Geometry: final body of the model. Coordinates: model frame, mm. A direction names the side the tool comes from. Coordinates: 2 decimals unless noted, no trailing zeros. Write each loop counter-clockwise with the first axis right and the second up, starting at its lowest first coordinate (ties: lowest second). Pieces come first, ordered by that corner, then holes. Notation, with made-up numbers: (-20, 89.25) - (38, 89.25) arc R12 ccw to (38, 96.25) - close; hole circle Ø2 at (5.25, 4). An arc over 180 degrees is marked (long way). Put each result on its own line as item: value.
```python
from build123d import *

# Parameters (mm, degrees)
F1_DEPTH  = 21
F2_W      = 22
F2_H      = 21
F3_DEPTH  = 4
F4_R      = 6.6
F4_R_2    = 1.35
F5_DEPTH  = 17.501
F6_R      = 1.8
F7_DEPTH  = 7
F8_R      = 4
F9_DEPTH  = 3
F10_R     = 1.35
F11_DEPTH = 12


# Not quite as in the source:
# - a feature names something its author has since deleted; it is built from what else it names


with BuildPart() as f1:
    # F0 (on Front) → F1 (new body)
    with BuildSketch(Plane.XZ):
        with BuildLine():
            Line((-9, -2.5), (-6.5, 0))
            Line((-6.5, 0), (-11, 0))
            Line((-11, 0), (-11, -5))
            Line((-11, -5), (-6.5, -5))
            Line((-6.5, -5), (-6.5, -39))
            Line((-6.5, -39), (6.5, -39))
            Line((6.5, -39), (6.5, -5))
            Line((6.5, -5), (11, -5))
            Line((11, -5), (11, 0))
            Line((11, 0), (6.5, 0))
            Line((6.5, 0), (9, -2.5))
            Line((9, -2.5), (0.75, -2.5))
            Line((0.75, -2.5), (0.75, -17.11916493))
            ThreePointArc((0.75, -17.11916493), (0, -20.9732145518), (-0.75, -17.11916493))
            Line((-0.75, -17.11916493), (-0.75, -2.5))
            Line((-0.75, -2.5), (-9, -2.5))
        make_face()
    extrude(amount=F1_DEPTH)

    # F2 (on face) → F3 (cut)
    with BuildSketch(Plane.XZ.offset(21)):
        with Locations((0, -10.5)):
            Rectangle(F2_W, F2_H)
    extrude(amount=-F3_DEPTH, mode=Mode.SUBTRACT)

    # F4 (on face) → F5 (cut, through all)
    with BuildSketch(Plane.YZ.offset(6.5)):
        with Locations((-8.5, -30)):
            Circle(F4_R)
        with Locations((-8.5, -9.5)):
            Circle(F4_R_2)
    extrude(amount=-F5_DEPTH, mode=Mode.SUBTRACT)

    # F6 (on face) → F7 (cut)
    with BuildSketch(Plane.YZ.offset(6.5)):
        with Locations((-8.5, -9.5)):
            Circle(F6_R)
    extrude(amount=-F7_DEPTH, mode=Mode.SUBTRACT)

    # F8 (on face) → F9 (cut)
    with BuildSketch(Plane.YZ.offset(6.5)):
        with Locations((-8.5, -9.5)):
            Circle(F8_R)
    extrude(amount=-F9_DEPTH, mode=Mode.SUBTRACT)

    # F10 (on face) → F11 (cut)
    with BuildSketch(Plane.XZ.offset(21)):
        with Locations((0, -30)):
            Circle(F10_R)
    extrude(amount=-F11_DEPTH, mode=Mode.SUBTRACT)


solid = f1.part
```
1. Section query B-B (x = 4.25). Return loops of the section in (y, z), then the cut area to 3 significant figures.
Answer below:
outline: (-21, -39) - (0, -39) - (0, -2.5) - (-17, -2.5) - (-17, -21) - (-21, -21) - close; hole circle Ø13.2 at (-8.5, -30); hole circle Ø8 at (-8.5, -9.5)
area: 505 mm²
2. Set-up query: faces 1 (the flat face through (-9, -8, -5)), 2 (the flat face through (3.5, -9.44, -11.22)), 3 (the flat face through (0, -19, -21)), 4 (the flat face through (9, -8, -5)). Return all of +Z, -Z, +X, -X, +Y, -Y with unobstructed straight access to the full face (end or side cutting, diameter ignored); none if empty.
Answer below:
face 1: -Z, -X, +Y, -Y
face 2: +X
face 3: +Z, +X, -X, -Y
face 4: -Z, +X, +Y, -Y
3. Ray query, probe 1 along Z at (x, y) = (2.1, -8.5); probe 2 along Z at (x, y) = (4.55, -8.5); probe 3 along X at (y, z) = (-5.25, -11.5). Return the intervals inside material, ascending. Write a range as from..to.
Answer below:
probe 1: z = -39..-36.6, -23.4..-11.3, -7.7..-2.5
probe 2: z = -39..-36.6, -23.4..-13.5, -5.5..-2.5
probe 3: x = -6.5..-0.75, 0.75..3.5
4. Pin query (flat end, axial travel): pin 1 Ø6.5 at (y, z) = (-9, -18.5) entering from +X; pin 2 Ø2.5 at (y, z) = (-8.5, -9.5) entering from -X; pin 3 Ø10 at (y, z) = (-3.5, -13) entering from -X; pin 4 Ø6 at (y, z) = (-8.5, -9.5) entering from +X. Return the tip coordinate at first contact, or that it passes through.
Answer below:
pin 1: stops at x = 6.5
pin 2: passes through
pin 3: stops at x = -6.5
pin 4: stops at x = 3.5
5. Section query A-A (y = -8.5). Count the separate pieces of the cut face and the enclosed holes in it, then the cut area to 3 significant figures.
Answer below:
separate pieces: 4
enclosed holes: 0
area: 258 mm²
6. Section query C-C (z = -13). Return loops of the section in (x, y).
Answer below:
outline: (-6.5, -17) - (-0.75, -17) - (-0.75, 0) - (-6.5, 0) - close; (0.75, -17) - (6.5, -17) - (6.5, -10.44) - (3.5, -10.44) - (3.5, -6.56) - (6.5, -6.56) - (6.5, 0) - (0.75, 0) - close
7. Mould query, pull axis Z, two halves, no side actions, for faces 5 (the flat face through (5, -8, -2.5)), 6 (the flat face through (-0.75, -8, -12)), 7 (the flat face through (9, -8, 0)). Classes: +Z half, -Z half, draft (parallel to the pull), parting line (faces both ways), or undercut.
Answer below:
face 5: undercut
face 6: draft
face 7: +Z half
8. Section query D-D (z = -30). Return loops of the section in (x, y).
Answer below:
outline: (-6.5, -21) - (-1.35, -21) - (-1.35, -15.1) - (-6.5, -15.1) - close; (-6.5, -1.9) - (6.5, -1.9) - (6.5, 0) - (-6.5, 0) - close; (1.35, -21) - (6.5, -21) - (6.5, -15.1) - (1.35, -15.1) - close
